Could you check a few things on this model? Use its own coordinates, in mm. A direction names the side the tool comes from. Give positions to 0.01 mm unless a question says otherwise; leave off trailing zeros. Order: outer loops, then holes, each group sorted by start corner. A loop starts at its lowest first (then second) coordinate and runs counter-clockwise, first axis right, second up. Notation, with made-up numbers: M 25.5,8.5 L 57.5,8.5 A23 ccw 57.5,35.5 Z; hole C -33,85 d3. An arc over 180 degrees is marked long. Return JSON: item names as keys, results as strings. Group by question number.
```python
from build123d import *

# Parameters (mm, degrees)
BOSS_EXTRUDE5_DEPTH   = 2.54
SKETCH1_14_W          = 78.53
SKETCH1_14_H          = 58.08
SKETCH1_14_W_2        = 73.45
SKETCH1_14_H_2        = 53
BOSS_EXTRUDE6_DEPTH   = 17.78
SKETCH1_15_R          = 1.778
BOSS_EXTRUDE7_DEPTH   = 20.32
BOSS_EXTRUDE7_2_DEPTH = 20.32
SKETCH1_16_W          = 22.699017595
SKETCH1_16_H          = 8.472740405
SKETCH1_16_W_2        = 23.825224437
SKETCH1_16_H_2        = 8.631081672
SKETCH1_16_R          = 1.778
BOSS_EXTRUDE8_DEPTH   = 12.7635
SKETCH2_W             = 19.346850656
SKETCH2_H             = 7.764196645
CUT_EXTRUDE1_DEPTH    = 2.54
FILLET1_R             = 2.54


with BuildPart() as part:
    # Sketch1 → Boss-Extrude5 (new body)
    with BuildSketch(Plane(origin=(0, 0, 0), x_dir=(1, 0, 0), z_dir=(0, 1, 0))):
        Polygon((13.927874743, 17.78199044), (13.927874743, 26.254730845), (-14.124090067, 26.254730845), (-14.124090067, 17.78199044), (-36.823107662, 17.78199044), (-36.823107662, -26.745269155), (-12.176172828, -26.745269155), (-12.176172828, -18.114187483), (11.649051609, -18.114187483), (11.649051609, -26.745269155), (36.626892338, -26.745269155), (36.626892338, 17.78199044), align=None)
    extrude(amount=BOSS_EXTRUDE5_DEPTH)

    # Sketch1<14> → Boss-Extrude6 (add)
    with BuildSketch(Plane(origin=(0, 0, 0), x_dir=(1, 0, 0), z_dir=(0, 1, 0))):
        with Locations((-0.098107662, -0.245269155)):
            Rectangle(SKETCH1_14_W, SKETCH1_14_H)
        with Locations((-0.098107662, -0.245269155)):
            Rectangle(SKETCH1_14_W_2, SKETCH1_14_H_2, mode=Mode.SUBTRACT)
    extrude(amount=BOSS_EXTRUDE6_DEPTH)



with BuildPart() as body_2:
    # Sketch1<15> → Boss-Extrude7 (new body)
    with BuildSketch(Plane(origin=(0, 0, 0), x_dir=(1, 0, 0), z_dir=(0, 1, 0))):
        with Locations(Location((-4.171215324, -23.247161493, 0), (0, 0, 270))):
            Circle(SKETCH1_15_R)
    extrude(amount=BOSS_EXTRUDE7_DEPTH)


with BuildPart() as body_3:
    # Sketch1<15> → Boss-Extrude7 2 (new body)
    with BuildSketch(Plane(origin=(0, 0, 0), x_dir=(1, 0, 0), z_dir=(0, 1, 0))):
        with Locations(Location((4.428784676, -23.247161493, 0), (0, 0, 270))):
            Circle(SKETCH1_15_R)
    extrude(amount=BOSS_EXTRUDE7_2_DEPTH)


with BuildPart() as part_1:
    add(part.part)

    add(body_2.part)  # Boss-Extrude8 merges body 2

    add(body_3.part)  # Boss-Extrude8 merges body 3
    # Sketch1<16> → Boss-Extrude8 (add)
    # profile 1 of 3: a face of its own
    with BuildSketch(Plane(origin=(0, 0, 0), x_dir=(1, 0, 0), z_dir=(0, 1, 0))):
        with Locations((25.277383541, 22.018360642)):
            Rectangle(SKETCH1_16_W, SKETCH1_16_H)
    # profile 2 of 3: a face of its own
    with BuildSketch(Plane(origin=(0, 0, 0), x_dir=(1, 0, 0), z_dir=(0, 1, 0))):
        with Locations((-25.473598865, 22.018360642)):
            Rectangle(SKETCH1_16_W, SKETCH1_16_H)
    # profile 3 of 3: a face of its own
    with BuildSketch(Plane(origin=(0, 0, 0), x_dir=(1, 0, 0), z_dir=(0, 1, 0))):
        with Locations((-0.263560609, -22.429728319)):
            Rectangle(SKETCH1_16_W_2, SKETCH1_16_H_2)
        with Locations((-4.171215324, -23.247161493)):
            Circle(SKETCH1_16_R, mode=Mode.SUBTRACT)
        with Locations((4.428784676, -23.247161493)):
            Circle(SKETCH1_16_R, mode=Mode.SUBTRACT)
    extrude(amount=BOSS_EXTRUDE8_DEPTH)

    # Sketch2 → Cut-Extrude1 (cut)
    with BuildSketch(Plane.ZY.offset(39.363107662)):
        with Locations((0.640618985, 7.290284295)):
            Rectangle(SKETCH2_W, SKETCH2_H)
    extrude(amount=-CUT_EXTRUDE1_DEPTH, mode=Mode.SUBTRACT)

    # Fillet1
    fillet1_edges = [part_1.edges().sort_by_distance(p)[0] for p in [
        (-39.363107662, 8.89, 29.285269155),
        (39.166892338, 8.89, 29.285269155),
        (39.166892338, 8.89, -28.794730845),
        (-39.363107662, 8.89, -28.794730845),
    ]]
    fillet(fillet1_edges, radius=FILLET1_R)


solid = part_1.part
```
1. For pin 1 (1.3 mm diameter, centred on x = -38, z = -2, fed in from +Y); pin 2 (4 mm diameter, centred on x = 29, z = 19, fed in from +Y); pin 3 (2 mm diameter, centred on x = -38.5, y = 7.5, fed in from -Z), each with a flat end and sliding along its axis, tell me the tip position at first contact or that it passes through.
2. Imagine slicing it at B-B, the plane y = 6.5. Please give me the cut outline in (x, z), plus the area to 3 significant figures.
3. If we mould it in two halves opening along X, with no side actions, what happens to faces 4 (the flat face through (-38, 3.408, 1)), 5 (the cylindrical face through (38.403, 9.014, 28.561)), 6 (the flat face through (-1, 13, 26.745)), 7 (the flat face through (-1, 12, -26.255))? For each: pulls with the +X half, pulls with the -X half, needs draft (parallel to the pull), parting line crosses it, or undercut.
4. Imagine slicing it at D-D, the plane z = 20. Please give me the cut outline in (x, y), plus the area to 3 significant figures.
5. Which directions (+Z, -Z, +X, -X, +Y, -Y) give clear straight access to the entire face, cutting with the end or side of a thin tool? Please do faces 1 (the flat face through (-38, 7, -9.033)), 2 (the flat face through (11.649, 8, 22)), 3 (the flat face through (-1, 9, -28.795)).
6. Imagine slicing it at C-C, the plane x = 0. Please give me the cut outline in (y, z).
7. Imagine slicing it at A-A, the plane z = -0.5. Please give me the cut outline in (x, y).
8. I need wall thicknesses on L1, parallel to Z at x = -30.5, y = 13.5; L2, parallel to Z at x = -6, y = 7.75; L3, parallel to X at y = 11.25, z = 19. Which ranges of each line are inside material? Lowest first, please. Write a range as from..to.
Values:
{
 "1": {"pin 1": "stops at y = 17.78", "pin 2": "stops at y = 2.54", "pin 3": "stops at z = -28.7"},
 "2": {"outline": "M -39.36,-26.25 A2.54 ccw -36.82,-28.79 L 36.63,-28.79 A2.54 ccw 39.17,-26.25 L 39.17,26.75 A2.54 ccw 36.63,29.29 L -36.82,29.29 A2.54 ccw -39.36,26.75 L -39.36,10.31 L -36.82,10.31 L -36.82,26.75 L -12.18,26.75 L -12.18,18.11 L 11.65,18.11 L 11.65,26.75 L 36.63,26.75 L 36.63,-17.78 L 13.93,-17.78 L 13.93,-26.25 L -14.12,-26.25 L -14.12,-17.78 L -36.82,-17.78 L -36.82,-9.03 L -39.36,-9.03 Z", "area": "1,200 mm²"},
 "3": {"face 4": "needs draft", "face 5": "pulls with the +X half", "face 6": "undercut", "face 7": "undercut"},
 "4": {"outline": "M -39.36,0 L 39.17,0 L 39.17,17.78 L 36.63,17.78 L 36.63,2.54 L 11.65,2.54 L 11.65,12.76 L -12.18,12.76 L -12.18,2.54 L -36.82,2.54 L -36.82,17.78 L -39.36,17.78 Z", "area": "520 mm²"},
 "5": {"face 1": "-X", "face 2": "+Y", "face 3": "-Z, +X, -X, +Y, -Y"},
 "6": {"outline": "M 0,-28.79 L 17.78,-28.79 L 17.78,-26.25 L 2.54,-26.25 L 2.54,18.11 L 12.76,18.11 L 12.76,26.75 L 17.78,26.75 L 17.78,29.29 L 0,29.29 Z"},
 "7": {"outline": "M -39.36,0 L 39.17,0 L 39.17,17.78 L 36.63,17.78 L 36.63,2.54 L -36.82,2.54 L -36.82,3.41 L -39.36,3.41 Z; M -39.36,11.17 L -36.82,11.17 L -36.82,17.78 L -39.36,17.78 Z"},
 "8": {"L1": "z = -28.79..-26.25, 26.75..29.29", "L2": "z = -28.79..-26.25, 18.11..29.29", "L3": "x = -39.36..-36.82, -12.18..11.65, 36.63..39.17"}
}
